The model under review builds one solid part; all positions refer to its coordinate system, in mm. A direction names the side the tool comes from. Coordinates: 2 decimals unless noted, no trailing zeros. Write each loop counter-clockwise with the first axis right and the second up, starting at its lowest first coordinate (ties: lowest second). Pieces come first, ordered by that corner, then holes. Notation, with made-up numbers: (55.25, 38.5) - (71.25, 38.5) arc R29 ccw to (71.25, 64.5) - close; hole circle Ø7 at (-4.5, 19.25). An arc over 180 degrees is marked (long way). Return JSON: item names as keys, results as strings. Group by question number.
(1) We need section A-A on z = -78.5. State the section outline as (x, y) points.
(2) For pin 1 Ø5 at (x, z) = (111.935, -273.49) entering from +Y; pin 2 Ø1 at (y, z) = (4.5, -196.5) entering from +X; pin 3 Ø5 at (y, z) = (26, -218.5) entering from -X; pin 4 Ø9 at (y, z) = (13, -304) entering from +X, all flat-tipped, find the tip position at first contact; note any pin that passes through.
(3) We need section D-D on x = 16.5. State the section outline as (y, z) points.
(4) Tool access review of faces 1 (the face through (318.87, 15, -45)), 2 (the face through (420.37, 15, -306)), 3 (the face through (0, 15, -45)): name each direction out of +Z, -Z, +X, -X, +Y, -Y from which nothing blocks a thin tool from reaching the whole face with its end or side.
(5) We need section B-B on x = 303.87. State the section outline as (y, z) points.
(6) To check wall thickness, follow L1, parallel to X at y = 13, z = -318.49 (3 decimals); L2, parallel to X at y = 15.25, z = -283.49 (3 decimals); L3, parallel to Z at x = 495.81, y = 13. State the ranges of each line that lie inside material, in increasing order. Write a range as from..to.
(7) Draft analysis for pull direction Z (two halves, no side actions). For faces 4 (the face through (-177.955, 14.79, -178.652)), 5 (the face through (-163.759, 14.79, -214.057)), 6 (the face through (-199.5, 15, -298)), 7 (the face through (441.307, 14.79, -146.941)), state which applies: released by +Z, released by -Z, zero draft, split by the parting line, or undercut.
(8) We need section C-C on y = 19.25. Give the number of separate pieces and of enclosed holes in the cut face, then the cut area to 3 significant figures.
```python
from build123d import *

# Parameters (mm, degrees)
SKETCH1_R           = 4.25
SKETCH1_R_2         = 25.1
SKETCH1_R_3         = 7
BOSS_EXTRUDE1_DEPTH = 30


with BuildPart() as part:
    # Sketch1 → Boss-Extrude1 (new body)
    with BuildSketch(Plane(origin=(0, 0, 0), x_dir=(1, 0, 0), z_dir=(0, 1, 0))):
        with BuildLine():
            Line((0, 0), (273.87, 0))
            Line((273.87, 0), (273.87, 88.502095305))
            ThreePointArc((273.87, 88.502095305), (296.37, 111.002095305), (318.87, 88.502095305))
            Line((318.87, 88.502095305), (318.87, 0))
            Line((318.87, 0), (592.74, 0))
            Line((592.74, 0), (592.74, 184.192095305))
            ThreePointArc((592.74, 184.192095305), (533.806093864, 226.410155161), (511.25, 295.307125341))
            Line((511.25, 295.307125341), (511.25, 333.742095305))
            ThreePointArc((511.25, 333.742095305), (508.321067812, 340.813163117), (501.25, 343.742095305))
            Line((501.25, 343.742095305), (430.37, 343.742095305))
            ThreePointArc((430.37, 343.742095305), (423.298932188, 340.813163117), (420.37, 333.742095305))
            Line((420.37, 333.742095305), (420.37, 278.472002111))
            ThreePointArc((420.37, 278.472002111), (303.87, 161.972002111), (187.37, 278.472002111))
            Line((187.37, 278.472002111), (187.37, 333.742095305))
            ThreePointArc((187.37, 333.742095305), (184.441067812, 340.813163117), (177.37, 343.742095305))
            Line((177.37, 343.742095305), (106.5, 343.742095305))
            ThreePointArc((106.5, 343.742095305), (99.428932188, 340.813163117), (96.5, 333.742095305))
            Line((96.5, 333.742095305), (96.5, 278.472002111))
            ThreePointArc((96.5, 278.472002111), (-20, 161.972002111), (-136.5, 278.472002111))
            Line((-136.5, 278.472002111), (-136.5, 333.742095305))
            ThreePointArc((-136.5, 333.742095305), (-139.428932188, 340.813163117), (-146.5, 343.742095305))
            Line((-146.5, 343.742095305), (-189.5, 343.742095305))
            ThreePointArc((-189.5, 343.742095305), (-196.571067812, 340.813163117), (-199.5, 333.742095305))
            Line((-199.5, 333.742095305), (-199.5, 260.976228759))
            ThreePointArc((-199.5, 260.976228759), (-177.402461095, 177.567779789), (-122.5, 111.002095305))
            Line((-122.5, 111.002095305), (-22.5, 111.002095305))
            ThreePointArc((-22.5, 111.002095305), (-6.590097423, 104.411997882), (0, 88.502095305))
            Line((0, 88.502095305), (0, 0))
        make_face()
        with Locations(Location((-188, 328.49, 0), (0, 0, 270))):
            Circle(SKETCH1_R, mode=Mode.SUBTRACT)
        with Locations(Location((-148, 328.49, 0), (0, 0, 270))):
            Circle(SKETCH1_R, mode=Mode.SUBTRACT)
        with Locations(Location((-188, 273.49, 0), (0, 0, 270))):
            Circle(SKETCH1_R, mode=Mode.SUBTRACT)
        with Locations(Location((-148, 273.49, 0), (0, 0, 270))):
            Circle(SKETCH1_R, mode=Mode.SUBTRACT)
        with Locations(Location((-168, 318.49, 0), (0, 0, 270))):
            Circle(SKETCH1_R, mode=Mode.SUBTRACT)
        with Locations(Location((-168, 283.49, 0), (0, 0, 270))):
            Circle(SKETCH1_R, mode=Mode.SUBTRACT)
        with Locations(Location((111.935, 328.49, 0), (0, 0, 270))):
            Circle(SKETCH1_R, mode=Mode.SUBTRACT)
        with Locations(Location((171.935, 328.49, 0), (0, 0, 270))):
            Circle(SKETCH1_R, mode=Mode.SUBTRACT)
        with Locations(Location((111.935, 273.49, 0), (0, 0, 270))):
            Circle(SKETCH1_R, mode=Mode.SUBTRACT)
        with Locations(Location((171.935, 273.49, 0), (0, 0, 270))):
            Circle(SKETCH1_R, mode=Mode.SUBTRACT)
        with Locations(Location((141.935, 318.49, 0), (0, 0, 270))):
            Circle(SKETCH1_R, mode=Mode.SUBTRACT)
        with Locations(Location((141.935, 283.49, 0), (0, 0, 270))):
            Circle(SKETCH1_R, mode=Mode.SUBTRACT)
        with Locations(Location((435.81, 328.49, 0), (0, 0, 270))):
            Circle(SKETCH1_R, mode=Mode.SUBTRACT)
        with Locations(Location((495.81, 328.49, 0), (0, 0, 270))):
            Circle(SKETCH1_R, mode=Mode.SUBTRACT)
        with Locations(Location((435.81, 273.49, 0), (0, 0, 270))):
            Circle(SKETCH1_R, mode=Mode.SUBTRACT)
        with Locations(Location((495.81, 273.49, 0), (0, 0, 270))):
            Circle(SKETCH1_R, mode=Mode.SUBTRACT)
        with Locations(Location((465.81, 318.49, 0), (0, 0, 270))):
            Circle(SKETCH1_R, mode=Mode.SUBTRACT)
        with Locations(Location((465.81, 283.49, 0), (0, 0, 270))):
            Circle(SKETCH1_R, mode=Mode.SUBTRACT)
        with Locations(Location((465.81, 71.5, 0), (0, 0, 270))):
            Circle(SKETCH1_R_2, mode=Mode.SUBTRACT)
        with Locations(Location((465.81, 141.5, 0), (0, 0, 270))):
            Circle(SKETCH1_R_2, mode=Mode.SUBTRACT)
        with Locations(Location((465.81, 211.5, 0), (0, 0, 270))):
            Circle(SKETCH1_R_2, mode=Mode.SUBTRACT)
        with Locations(Location((465.81, 174.25, 0), (0, 0, 270))):
            Circle(SKETCH1_R, mode=Mode.SUBTRACT)
        with Locations(Location((453.27711759, 171.75705469, 0), (0, 0, 270))):
            Circle(SKETCH1_R, mode=Mode.SUBTRACT)
        with Locations(Location((442.652252916, 164.657747084, 0), (0, 0, 270))):
            Circle(SKETCH1_R, mode=Mode.SUBTRACT)
        with Locations(Location((435.55294531, 154.03288241, 0), (0, 0, 270))):
            Circle(SKETCH1_R, mode=Mode.SUBTRACT)
        with Locations(Location((433.06, 141.5, 0), (0, 0, 270))):
            Circle(SKETCH1_R, mode=Mode.SUBTRACT)
        with Locations(Location((453.27711759, 111.24294531, 0), (0, 0, 270))):
            Circle(SKETCH1_R, mode=Mode.SUBTRACT)
        with Locations(Location((442.652252916, 118.342252916, 0), (0, 0, 270))):
            Circle(SKETCH1_R, mode=Mode.SUBTRACT)
        with Locations(Location((435.55294531, 128.96711759, 0), (0, 0, 270))):
            Circle(SKETCH1_R, mode=Mode.SUBTRACT)
        with Locations(Location((465.81, 108.75, 0), (0, 0, 270))):
            Circle(SKETCH1_R, mode=Mode.SUBTRACT)
        with Locations(Location((478.34288241, 111.24294531, 0), (0, 0, 270))):
            Circle(SKETCH1_R, mode=Mode.SUBTRACT)
        with Locations(Location((488.967747084, 118.342252916, 0), (0, 0, 270))):
            Circle(SKETCH1_R, mode=Mode.SUBTRACT)
        with Locations(Location((496.06705469, 128.96711759, 0), (0, 0, 270))):
            Circle(SKETCH1_R, mode=Mode.SUBTRACT)
        with Locations(Location((498.56, 141.5, 0), (0, 0, 270))):
            Circle(SKETCH1_R, mode=Mode.SUBTRACT)
        with Locations(Location((496.06705469, 154.03288241, 0), (0, 0, 270))):
            Circle(SKETCH1_R, mode=Mode.SUBTRACT)
        with Locations(Location((488.967747084, 164.657747084, 0), (0, 0, 270))):
            Circle(SKETCH1_R, mode=Mode.SUBTRACT)
        with Locations(Location((478.34288241, 171.75705469, 0), (0, 0, 270))):
            Circle(SKETCH1_R, mode=Mode.SUBTRACT)
        with Locations(Location((141.935, 161.5, 0), (0, 0, 270))):
            Circle(SKETCH1_R_2, mode=Mode.SUBTRACT)
        with Locations(Location((141.935, 91.5, 0), (0, 0, 270))):
            Circle(SKETCH1_R_2, mode=Mode.SUBTRACT)
        with Locations(Location((-159.5, 208.502095305, 0), (0, 0, 270))):
            Circle(SKETCH1_R_3, mode=Mode.SUBTRACT)
    extrude(amount=BOSS_EXTRUDE1_DEPTH)


solid = part.part
```
Ans:
{
 "1": {"outline": "(0, 0) - (120.46, 0) - (120.46, 30) - (0, 30) - close; (163.41, 0) - (273.87, 0) - (273.87, 30) - (163.41, 30) - close; (318.87, 0) - (441.71, 0) - (441.71, 30) - (318.87, 30) - close; (489.91, 0) - (592.74, 0) - (592.74, 30) - (489.91, 30) - close"},
 "2": {"pin 1": "through", "pin 2": "x = 566.84", "pin 3": "x = -193.71", "pin 4": "x = 511.25"},
 "3": {"outline": "(0, -167.84) - (30, -167.84) - (30, 0) - (0, 0) - close"},
 "4": {"face 1": "+Z, +Y, -Y", "face 2": "-Z, +Y, -Y", "face 3": "+Z, -X, +Y, -Y"},
 "5": {"outline": "(0, -161.97) - (30, -161.97) - (30, -109.72) - (0, -109.72) - close"},
 "6": {"L1": "-199.5..-172.25, -163.75..-136.5, 96.5..137.685, 146.185..187.37, 420.37..461.56, 470.06..511.25", "L2": "-199.5..-172.25, -163.75..-136.5, 96.5..137.685, 146.185..187.37, 420.37..461.56, 470.06..511.851", "L3": "-343.74..-332.74, -324.24..-277.74, -269.24..-158.28, -149.79..-144.74, -138.26..-133.21, -124.72..0"},
 "7": {"face 4": "released by +Z", "face 5": "undercut", "face 6": "zero draft", "face 7": "undercut"},
 "8": {"separate pieces": "1", "enclosed holes": "40", "area": "146,000 mm²"}
}
